Check sheet for the modelled part. Datum: model origin and axes. Units: mm. A direction names the side the tool comes from. Coordinates: 2 decimals unless noted, no trailing zeros. Loops run counter-clockwise (first coordinate to the right, second up) from the corner with the lowest first, then second, coordinate; pieces in that order, holes last. Notation, with made-up numbers: M 24,25 L 37,25 A24 ccw 37,54 Z; hole C 67.5,0.5 d7. An arc over 180 degrees is marked long. Write each question's results on one line, items separated by ' | '. Start each with the question number.
from build123d import *

# Parameters (mm, degrees)
F0_R     = 1.95
F1_DEPTH = 4.8
F0_W     = 15
F0_H     = 4
F2_DEPTH = 20.15
F0_H_2   = 10.6
F0_R_2   = 4.25
F0_R_3   = 2.25
F3_DEPTH = 30.15
F4_DEPTH = 3.4
F5_DEPTH = 3.6
F6_DEPTH = 3.4


with BuildPart() as f1:
    # F0 (on Front) → F1 (new body)
    with BuildSketch(Plane.XZ):
        Polygon((7.5, 21.35), (-7.5, 21.35), (-7.5, -21.35), (7.5, -21.35), (7.5, 14), align=None)
        with Locations((-3.25, -19)):
            Circle(F0_R, mode=Mode.SUBTRACT)
        with BuildLine():
            Line((39.75, 24), (7.5, 24))
            Line((7.5, 24), (7.5, 21.35))
            Line((7.5, 21.35), (7.5, 14))
            Line((7.5, 14), (39.75, 14))
            ThreePointArc((39.75, 14), (44.75, 19), (39.75, 24))
        make_face()
        with Locations((39.75, 19)):
            Circle(F0_R, mode=Mode.SUBTRACT)
    extrude(amount=F1_DEPTH)

    # F0 (on Front) → F2 (join)
    with BuildSketch(Plane.XZ):
        Polygon((7.5, 24), (7.5, 25.35), (-7.5, 25.35), (-7.5, 21.35), (7.5, 21.35), align=None)
        with Locations((0, -23.35)):
            Rectangle(F0_W, F0_H)
    extrude(amount=F2_DEPTH)

    # F0 (on Front) → F3 (join)
    with BuildSketch(Plane.XZ):
        with Locations((0, 30.65)):
            Rectangle(F0_W, F0_H_2)
        with Locations((0, 30.05)):
            Circle(F0_R_2, mode=Mode.SUBTRACT)
        with Locations((0, 30.05)):
            Circle(F0_R_2)
        with Locations((0, 30.05)):
            Circle(F0_R_3, mode=Mode.SUBTRACT)
        with Locations((0, -30.65)):
            Rectangle(F0_W, F0_H_2)
        with Locations((0, -30.05)):
            Circle(F0_R_2, mode=Mode.SUBTRACT)
        with Locations((0, -30.05)):
            Circle(F0_R_2)
        with Locations((0, -30.05)):
            Circle(F0_R_3, mode=Mode.SUBTRACT)
    extrude(amount=F3_DEPTH)

    # F0 (on Front) → F4 (cut)
    with BuildSketch(Plane.XZ):
        with Locations((0, -30.05)):
            Circle(F0_R_2)
        with Locations((0, -30.05)):
            Circle(F0_R_3, mode=Mode.SUBTRACT)
        with Locations((0, 30.05)):
            Circle(F0_R_2)
        with Locations((0, 30.05)):
            Circle(F0_R_3, mode=Mode.SUBTRACT)
    extrude(amount=F4_DEPTH, mode=Mode.SUBTRACT)

    # F0 (on Front) → F5 (join)
    with BuildSketch(Plane.XZ):
        with Locations((0, 30.05)):
            Circle(F0_R_3)
        with Locations((0, -30.05)):
            Circle(F0_R_3)
    extrude(amount=F5_DEPTH)

    # F0 (on Front) → F6 (cut)
    with BuildSketch(Plane.XZ):
        with Locations((0, -30.05)):
            Circle(F0_R_3)
        with Locations((0, 30.05)):
            Circle(F0_R_3)
    extrude(amount=F6_DEPTH, mode=Mode.SUBTRACT)


solid = f1.part
1) Section check D-D (x = 0). Enter the section's corners in (y, z).
2) Set-up check for faces 4 (the flat face through (23, -2, 14)), 5 (the flat face through (0, -25, 25.35)), 6 (the cylindrical face through (-0.92, -1.68, -34.2)), 7 (the flat face through (0, -3.6, -30)): record each of +Z, -Z, +X, -X, +Y, -Y from which the full face is reachable in a straight line by a thin tool's end or side.
3) Gauge pin test, flat ends, axial feed: P1, Ø1.5, axis at x = -0.5, z = -22, coming from the -Y side; P2, Ø2.5, axis at x = 1, z = -28, coming from the +Y side; P3, Ø12, axis at y = -11.5, z = -8, coming from the +X side; P4, Ø2.5, axis at x = 0, z = 30.05, coming from the -Y side. Record the tip position at first contact, or that the pin passes through.
4) Section check B-B (z = -19). Enter the section's corners in (x, y), then the cut area to 3 significant figures.
5) Section check A-A (y = -1.5). Enter the section's corners in (x, z).
6) Section check C-C (y = -26.5). Enter the section's corners in (x, z), then the cut area to 3 significant figures.
7) Release check for a two-part mould opening along Z. For faces 1 (the flat face through (0, -25, -25.35)), 2 (the flat face through (0, -15, 35.95)), 3 (the flat face through (7, 0, 1)) record: +Z half, -Z half, draft (parallel to the pull), parting line (faces both ways), or undercut.
8) Thickness scan on probe 1 along Z at (x, y) = (0, -2.5); probe 2 along Z at (x, y) = (0, -19.5); probe 3 along Z at (x, y) = (-2, -18). Record the ranges inside material, lowest first.
Return value:
1) outline: M -30.15,-35.95 L 0,-35.95 L 0,-34.3 L -3.4,-34.3 L -3.4,-25.8 L 0,-25.8 L 0,25.8 L -3.4,25.8 L -3.4,34.3 L 0,34.3 L 0,35.95 L -30.15,35.95 L -30.15,32.3 L -3.6,32.3 L -3.6,27.8 L -30.15,27.8 L -30.15,25.35 L -20.15,25.35 L -20.15,21.35 L -4.8,21.35 L -4.8,-21.35 L -20.15,-21.35 L -20.15,-25.35 L -30.15,-25.35 L -30.15,-27.8 L -3.6,-27.8 L -3.6,-32.3 L -30.15,-32.3 Z
2) face 4: -Z, +X, +Y, -Y | face 5: +X, -X, -Y | face 6: +Y | face 7: -Y
3) P1: stops at y = -20.15 | P2: stops at y = -3.4 | P3: passes through | P4: stops at y = -3.6
4) outline: M -7.5,-4.8 L -5.2,-4.8 L -5.2,0 L -7.5,0 Z; M -1.3,-4.8 L 7.5,-4.8 L 7.5,0 L -1.3,0 Z | area: 53.3 mm2
5) outline: M -7.5,-35.95 L 7.5,-35.95 L 7.5,14 L 39.75,14 A5 ccw 39.75,24 L 7.5,24 L 7.5,35.95 L -7.5,35.95 Z; hole C -3.25,-19 d3.9; hole C 0,-30.05 d8.5; hole C 0,30.05 d8.5; hole C 39.75,19 d3.9
6) outline: M -7.5,-35.95 L 7.5,-35.95 L 7.5,-25.35 L -7.5,-25.35 Z; M -7.5,25.35 L 7.5,25.35 L 7.5,35.95 L -7.5,35.95 Z; hole C 0,-30.05 d4.5; hole C 0,30.05 d4.5 | area: 286 mm2
7) face 1: undercut | face 2: +Z half | face 3: draft
8) probe 1: z = -35.95 to -34.3, -25.8 to 25.8, 34.3 to 35.95 | probe 2: z = -35.95 to -32.3, -27.8 to -21.35, 21.35 to 27.8, 32.3 to 35.95 | probe 3: z = -35.95 to -31.08, -29.02 to -21.35, 21.35 to 29.02, 31.08 to 35.95
